Autodesk Inventor part; units mm, degrees
ref_plane "YZ Plane" through (0, 0, 0) normal (1, 0, 0) x (0, 1, 0)
ref_plane "XZ Plane" through (0, 0, 0) normal (0, 1, 0) x (-1, 0, 0)
ref_plane "XY Plane" through (0, 0, 0) normal (0, 0, 1) x (1, 0, 0)
sketch "Sketch3" plane through (0, 0, 0) normal (0, 1, 0) x (-1, 0, 0)
  line L0 (72.5, 90) -> (-72.5, 90)
  line L1 (-72.5, 90) -> (-72.5, -90)
  line L2 (-72.5, -90) -> (72.5, -90)
  line L3 (72.5, -90) -> (72.5, 90)
  line L4 (72.5, 90) -> (-72.5, -90) construction
  line L5 (-72.5, 90) -> (72.5, -90) construction
  point P0 (0, 0)
  dimension "d7" = 145
  dimension "d8" = 180
extrude "Extrusion3" add sketch "Sketch3" along normal blind 5
sketch "Sketch4" plane through (0, 5, 0) normal (0, 1, 0) x (1, 0, 0)
  line L0 (23.935, -64) -> (72.5, -64)
  line L1 (72.5, -64) -> (72.5, -26.408)
  line L2 (72.5, -26.408) -> (23.935, -26.408)
  line L3 (23.935, -26.408) -> (23.935, -64)
  line L4 (23.935, -64) -> (72.5, -26.408) construction
  line L5 (72.5, -64) -> (23.935, -26.408) construction
  line L6 (72.5, -90) -> (72.5, 90)
  line L7 (-72.5, -90) -> (72.5, -90)
  line L8 (-72.5, -64) -> (-23.935, -64)
  line L9 (-23.935, -64) -> (-23.935, -26.408)
  line L10 (-23.935, -26.408) -> (-72.5, -26.408)
  line L11 (-72.5, -26.408) -> (-72.5, -64)
  line L12 (-72.5, -64) -> (-23.935, -26.408) construction
  line L13 (-23.935, -64) -> (-72.5, -26.408) construction
  line L14 (-72.5, 90) -> (-72.5, -90)
  point P0 (0, 0)
  point P1 (48.2175, -45.204)
  point P2 (-48.2175, -45.204)
  dimension "d11" = 48.565
  dimension "d12" = 37.592
  dimension "d13" = 0
  dimension "d14" = 26
  dimension "d20" = 48.565
  dimension "d21" = 37.592
  dimension "d22" = 0
  dimension "d23" = 26
extrude "Extrusion4" cut sketch "Sketch4" against normal blind 2
sketch "Sketch5" plane through (0, 3, 0) normal (0, 1, 0) x (1, 0, 0)
  circle A0 centre (66.797, -60.825) radius 1.588
  line L0 (72.5, -26.408) -> (72.5, -64)
  line L1 (72.5, -64) -> (23.935, -64)
  circle A1 centre (60.447, -60.825) radius 1.588
  circle A2 centre (54.097, -60.825) radius 1.588
  circle A3 centre (47.747, -60.825) radius 1.588
  circle A4 centre (41.397, -60.825) radius 1.588
  circle A5 centre (35.047, -60.825) radius 1.588
  circle A6 centre (28.697, -60.825) radius 1.588
  circle A7 centre (66.797, -29.583) radius 1.588
  circle A8 centre (60.447, -29.583) radius 1.588
  circle A9 centre (54.097, -29.583) radius 1.588
  circle A10 centre (47.747, -29.583) radius 1.588
  circle A11 centre (41.397, -29.583) radius 1.588
  circle A12 centre (35.047, -29.583) radius 1.588
  circle A13 centre (28.697, -29.583) radius 1.588
  circle A14 centre (-66.797, -60.825) radius 1.588
  line L2 (-23.935, -64) -> (-72.5, -64)
  line L3 (-72.5, -64) -> (-72.5, -26.408)
  circle A15 centre (-60.447, -60.825) radius 1.588
  circle A16 centre (-54.097, -60.825) radius 1.588
  circle A17 centre (-47.747, -60.825) radius 1.588
  circle A18 centre (-41.397, -60.825) radius 1.588
  circle A19 centre (-35.047, -60.825) radius 1.588
  circle A20 centre (-28.697, -60.825) radius 1.588
  circle A21 centre (-66.797, -29.583) radius 1.588
  circle A22 centre (-60.447, -29.583) radius 1.588
  circle A23 centre (-54.097, -29.583) radius 1.588
  circle A24 centre (-47.747, -29.583) radius 1.588
  circle A25 centre (-41.397, -29.583) radius 1.588
  circle A26 centre (-35.047, -29.583) radius 1.588
  circle A27 centre (-28.697, -29.583) radius 1.588
  point P0 (0, 0)
  dimension "d24" = 3.176
  dimension "d25" = 5.703
  dimension "d26" = 3.175
  dimension "d30" = 6.35
  dimension "d33" = 31.242
  dimension "d36" = 3.176
  dimension "d37" = 3.175
  dimension "d38" = 5.703
  dimension "d41" = 6.35
  dimension "d44" = 31.242
extrude "Extrusion5" cut sketch "Sketch5" against normal through all
sketch "Sketch6" plane through (0, 5, 0) normal (0, 1, 0) x (1, 0, 0)
  line L0 (42.5, 32.6926) -> (52.5, 32.6926)
  line L1 (52.5, 32.6926) -> (52.5, 37.6926)
  line L2 (52.5, 37.6926) -> (42.5, 37.6926)
  line L3 (42.5, 37.6926) -> (42.5, 32.6926)
  line L4 (42.5, 32.6926) -> (52.5, 37.6926) construction
  line L5 (52.5, 32.6926) -> (42.5, 37.6926) construction
  line L6 (72.5, -26.408) -> (72.5, 90)
  line L7 (-52.5, 32.6926) -> (-42.5, 32.6926)
  line L8 (-42.5, 32.6926) -> (-42.5, 37.6926)
  line L9 (-42.5, 37.6926) -> (-52.5, 37.6926)
  line L10 (-52.5, 37.6926) -> (-52.5, 32.6926)
  line L11 (-52.5, 32.6926) -> (-42.5, 37.6926) construction
  line L12 (-42.5, 32.6926) -> (-52.5, 37.6926) construction
  line L13 (-72.5, 90) -> (-72.5, -26.408)
  line L14 (-52.5, -15.3074) -> (-42.5, -15.3074)
  line L15 (-42.5, -15.3074) -> (-42.5, -12.3074)
  line L16 (-42.5, -12.3074) -> (-52.5, -12.3074)
  line L17 (-52.5, -12.3074) -> (-52.5, -15.3074)
  line L18 (-52.5, -15.3074) -> (-42.5, -12.3074) construction
  line L19 (-42.5, -15.3074) -> (-52.5, -12.3074) construction
  line L20 (42.5, -15.3074) -> (52.5, -15.3074)
  line L21 (52.5, -15.3074) -> (52.5, -12.3074)
  line L22 (52.5, -12.3074) -> (42.5, -12.3074)
  line L23 (42.5, -12.3074) -> (42.5, -15.3074)
  line L24 (42.5, -15.3074) -> (52.5, -12.3074) construction
  line L25 (52.5, -15.3074) -> (42.5, -12.3074) construction
  arc A0 (-42.5, 37.6926) -> (-52.5, 37.6926) centre (-47.5, 37.6926) ccw
  arc A1 (52.5, 37.6926) -> (42.5, 37.6926) centre (47.5, 37.6926) ccw
  line L26 (-72.5, -26.408) -> (-23.935, -26.408)
  line L27 (23.935, -26.408) -> (72.5, -26.408)
  point P0 (0, 0)
  point P1 (47.5, 35.1926)
  point P2 (-47.5, 35.1926)
  point P3 (-47.5, -13.8074)
  point P4 (47.5, -13.8074)
  dimension "d49" = 10
  dimension "d50" = 5
  dimension "d51" = 20
  dimension "d52" = 10
  dimension "d53" = 5
  dimension "d54" = 20
  dimension "d57" = 10
  dimension "d58" = 3
  dimension "d59" = 10
  dimension "d60" = 3
  dimension "d61" = 45
  dimension "d84" = 11.1006
  dimension "d85" = 11.1006
extrude "Extrusion6" add sketch "Sketch6" along normal blind 24
sketch "Sketch7" plane through (0, 5, 0) normal (0, 1, 0) x (1, 0, 0)
  circle A0 centre (62.5, -80) radius 2.5
  line L0 (72.5, -90) -> (72.5, -64)
  line L1 (-72.5, -90) -> (72.5, -90)
  circle A1 centre (-62.5, -80) radius 2.5
  line L2 (-72.5, -64) -> (-72.5, -90)
  circle A2 centre (-39.5, -20.408) radius 2.5
  line L3 (-42.5, -15.3074) -> (-42.5, -12.3074)
  line L4 (-72.5, -26.408) -> (-23.935, -26.408)
  circle A3 centre (39.5, -20.408) radius 2.5
  line L5 (42.5, -12.3074) -> (42.5, -15.3074)
  line L6 (23.935, -26.408) -> (72.5, -26.408)
  line L7 (52.5, 35.6926) -> (42.5, 35.6926)
  circle A4 centre (39.5, -20.408) radius 4
  circle A5 centre (-39.5, -20.408) radius 4
  circle A6 centre (-62.5, -80) radius 4
  circle A7 centre (62.5, -80) radius 4
  circle A8 centre (-10, 53.3) radius 2.5
  line L8 (72.5, 90) -> (-72.5, 90)
  circle A9 centre (10, 53.3) radius 2.5
  circle A10 centre (0, -82.5) radius 2.5
  circle A11 centre (-40, -82.5) radius 2.5
  circle A12 centre (40, -82.5) radius 2.5
  point P0 (0, 0)
  point P1 (52.5, 37.6926)
  point P2 (42.5, 37.6926)
  point P3 (0, 90)
  point P4 (0, 90)
  point P5 (0, -90)
  dimension "d63" = 5
  dimension "d64" = 10
  dimension "d65" = 10
  dimension "d66" = 5
  dimension "d67" = 10
  dimension "d68" = 10
  dimension "d69" = 5
  dimension "d70" = 3
  dimension "d71" = 6
  dimension "d72" = 5
  dimension "d73" = 3
  dimension "d74" = 6
  dimension "d80" = 1.5
  dimension "d81" = 1.5
  dimension "d82" = 1.5
  dimension "d83" = 1.5
  dimension "d90" = 5
  dimension "d91" = 36.7
  dimension "d92" = 10
  dimension "d93" = 5
  dimension "d94" = 10
  dimension "d96" = 5
  dimension "d97" = 7.5
  dimension "d98" = 5
  dimension "d99" = 40
  dimension "d100" = 5
  dimension "d101" = 40
extrude "Extrusion7" cut sketch "Sketch7" against normal through all contours A0 | A1 | A2 | A3 | A8 | A9 | A10 | A11 | A12
sketch "Sketch8" plane through (0, 29, 0) normal (0, 1, 0) x (1, 0, 0)
  line L0 (-42.5, 32.6926) -> (-52.5, 32.6926)
  line L1 (-47.5, 32.6926) -> (-47.5, 42.6926)
  arc A0 (-42.5, 37.6926) -> (-52.5, 37.6926) centre (-47.5, 37.6926) ccw
  line L2 (42.5, 32.6926) -> (52.5, 32.6926)
  line L3 (47.5, 32.6926) -> (47.5, 42.6926)
  arc A1 (52.5, 37.6926) -> (42.5, 37.6926) centre (47.5, 37.6926) ccw
  circle A2 centre (47.5, 37.6926) radius 2.5
  circle A3 centre (-47.5, 37.6926) radius 2.5
  point P0 (0, 0)
  dimension "d86" = 5
  dimension "d87" = 5
extrude "Extrusion8" cut sketch "Sketch8" against normal blind 10
fillet "Fillet1" radius 6 4 edges at (72.5, 2.5, 90) (-72.5, 2.5, 90) (-72.5, 2.5, -90) (72.5, 2.5, -90)
properties part number "chasis"
Work out the finished part from the listing and answer in its coordinate system (mm). A direction names the side the tool comes from. Round coordinates to 2 decimals unless told otherwise and drop trailing zeros. Write each loop counter-clockwise with the first axis right and the second up, starting at its lowest first coordinate (ties: lowest second). Pieces come first, ordered by that corner, then holes. Notation, with made-up numbers: (3, -17) -> (16, -17) arc R9 cw to (16, -6) -> close; hole circle Ø7 at (55, -27.75). An arc over 180 degrees is marked (long way). Answer as CSV lines item,"result". Start each with the question number.
(1) The mould has two halves that part along X. Classify faces 1 (the flat face through (47, 17, 15.307)), 2 (the cylindrical face through (-47.61, 16.83, -42.69)), 3 (the cylindrical face through (70.789, 2.535, -88.196)): +X half, -X half, draft (parallel to the pull), parting line (faces both ways), or undercut.
(2) The part is cut by section C-C, the plane x = -10. Give the vertices of the cut face in (y, z), then the cut area to 3 significant figures.
(3) Each of these flat-tipped pins is pushed along its axis until it touches: pin 1 (4 mm diameter, centred on x = -47.747, z = 29.583, fed in from +Y); pin 2 (4 mm diameter, centred on x = -47.5, z = -37.69, fed in from +Y); pin 3 (0.9 mm diameter, centred on y = 19, z = 14, fed in from -X); pin 4 (4 mm diameter, centred on x = -62.5, z = 80, fed in from +Y). Where does it stop, or does it pass through?
(4) The part is cut by section B-B, the plane z = 49.5. Give the vertices of the cut face in (x, y) (3 decimals), then the cut area to 3 significant figures.
(5) The part is cut by section A-A, the plane y = 25. Give the vertices of the cut face in (x, z), then the cut area to 3 significant figures.
(6) The part is cut by section D-D, the plane y = 15.5. Give the vertices of the cut face in (x, z), then the cut area to 3 significant figures.
(7) Find the intervals of material crossed by probe 1 along Z at (x, y) = (-40, 3.25); probe 2 along Z at (x, y) = (-52, 22.5); probe 3 along Y at (x, z) = (46, -59.5), in increasing order.
(8) A tool of negligible diameter and unlimited length cuts with its end or side. For faces 4 (the flat face through (47, 19, -38)), 5 (the flat face through (-48, 17, -32.693)), 6 (the flat face through (48, 3, 45)), from which of +Z, -Z, +X, -X, +Y, -Y can it reach the whole face along a straight path? Write none if from no direction.
Output values:
1,face 1,"draft"
1,face 2,"undercut"
1,face 3,"+X half"
2,outline,"(0, -90) -> (5, -90) -> (5, -55.8) -> (0, -55.8) -> close; (0, -50.8) -> (5, -50.8) -> (5, 90) -> (0, 90) -> close"
2,area,"875 mm²"
3,pin 1,"stops at y = 3"
3,pin 2,"stops at y = 19"
3,pin 3,"stops at x = -52.5"
3,pin 4,"passes through"
4,outline,"(-72.5, 0) -> (72.5, 0) -> (72.5, 3) -> (23.935, 3) -> (23.935, 5) -> (-23.935, 5) -> (-23.935, 3) -> (-72.5, 3) -> close"
4,area,"531 mm²"
5,outline,"(-52.5, -37.69) arc R5 ccw to (-42.5, -37.69) -> (-42.5, -32.69) -> (-52.5, -32.69) -> close; (-52.5, 12.31) -> (-42.5, 12.31) -> (-42.5, 15.31) -> (-52.5, 15.31) -> close; (42.5, -37.69) arc R5 ccw to (52.5, -37.69) -> (52.5, -32.69) -> (42.5, -32.69) -> close; (42.5, 12.31) -> (52.5, 12.31) -> (52.5, 15.31) -> (42.5, 15.31) -> close; hole circle Ø5 at (-47.5, -37.69); hole circle Ø5 at (47.5, -37.69)"
5,area,"199 mm²"
6,outline,"(-52.5, -37.69) arc R5 ccw to (-42.5, -37.69) -> (-42.5, -32.69) -> (-52.5, -32.69) -> close; (-52.5, 12.31) -> (-42.5, 12.31) -> (-42.5, 15.31) -> (-52.5, 15.31) -> close; (42.5, -37.69) arc R5 ccw to (52.5, -37.69) -> (52.5, -32.69) -> (42.5, -32.69) -> close; (42.5, 12.31) -> (52.5, 12.31) -> (52.5, 15.31) -> (42.5, 15.31) -> close"
6,area,"239 mm²"
7,probe 1,"z = -90 to 17.96, 22.86 to 26.41, 64 to 80, 85 to 90"
7,probe 2,"z = -39.87 to -32.69, 12.31 to 15.31"
7,probe 3,"y = 0 to 5"
8,face 4,"+Y"
8,face 5,"+X, -X, +Y"
8,face 6,"+X, +Y"
